```python
from build123d import *

# Parameters (mm, degrees)
CYLINDER081_R     = 13.5
CYLINDER081_DEPTH = 20
CYLINDER080_R     = 15.7
CYLINDER080_DEPTH = 14
CYLINDER083_R     = 11
CYLINDER083_DEPTH = 1
CYLINDER082_R     = 15
CYLINDER082_DEPTH = 1


with BuildPart() as internal_border:
    # Cylinder081 → Cylinder081 (new body)
    with BuildSketch(Plane.XY):
        Circle(CYLINDER081_R)
    extrude(amount=CYLINDER081_DEPTH)


with BuildPart() as adapter_tube_cut:
    # Cylinder080 → Cylinder080 (new body)
    with BuildSketch(Plane.XY):
        Circle(CYLINDER080_R)
    extrude(amount=CYLINDER080_DEPTH)

    # Cut023016: cut internal border
    add(internal_border.part, mode=Mode.SUBTRACT)


with BuildPart() as top_plate_hole:
    # Cylinder083 → Cylinder083 (new body)
    with BuildSketch(Plane.XY):
        Circle(CYLINDER083_R)
    extrude(amount=CYLINDER083_DEPTH)


with BuildPart() as eyepiece_adapter_fusion:
    # Cylinder082 → Cylinder082 (new body)
    with BuildSketch(Plane.XY):
        Circle(CYLINDER082_R)
    extrude(amount=CYLINDER082_DEPTH)

    # Cut023015: cut top plate hole
    add(top_plate_hole.part, mode=Mode.SUBTRACT)

    # Fusion057: union adapter tube cut
    add(adapter_tube_cut.part)


solid = eyepiece_adapter_fusion.part
```
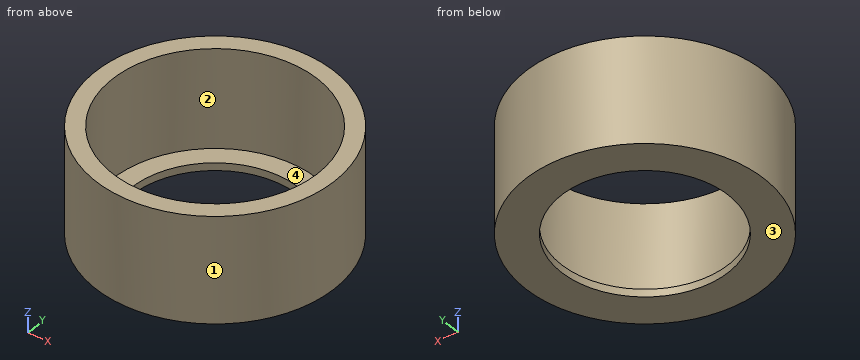
Verification items for the finished model (mm, model axes). Face numbers are marked on the shaded views. Coordinates: 2 decimals unless noted, no trailing zeros. Order: outer loops, then holes, each group sorted by start corner. A loop starts at its lowest first (then second) coordinate and runs counter-clockwise, first axis right, second up. Notation, with made-up numbers: (-21, 71.5) -> (12, 71.5) arc R21 cw to (12, 109.5) -> close; hole circle Ø4 at (56.25, -31.5). An arc over 180 degrees is marked (long way). Answer as CSV lines item,"result". Start each with the question number.
1) Cross-section at D-D, the plane y = -12. Record the boundary of the cut face in (x, z), then the cut area to 3 significant figures.
2) Gauge pin test, flat ends, axial feed: pin 1 Ø3 at (y, z) = (12.5, 2.5) entering from -X; pin 2 Ø8 at (y, z) = (-10, 7.5) entering from +X; pin 3 Ø2 at (x, z) = (8.5, 11.5) entering from +Y. Record the tip position at first contact, or that the pin passes through.
3) Cross-section at C-C, the plane z = 9. Record the boundary of the cut face in (x, y).
4) Release check for a two-part mould opening along X. For the marked faces 1, 2, 3 and 4 record: released by +X, released by -X, zero draft, split by the parting line, or undercut.
5) Cross-section at A-A, the plane y = 0. Record the boundary of the cut face in (x, z).
6) Material ranges on L1, parallel to Y at x = 0, z = 5.5; L2, parallel to Y at x = 0, z = 0.7; L3, parallel to Z at x = 7, y = -9, recorded low to high. Write a range as [from, to].
Conclusion:
1,outline,"(-10.12, 0) -> (10.12, 0) -> (10.12, 14) -> (6.18, 14) -> (6.18, 1) -> (-6.18, 1) -> (-6.18, 14) -> (-10.12, 14) -> close"
1,area,"123 mm²"
2,pin 1,"stops at x = -11.2"
2,pin 2,"stops at x = 14.51"
2,pin 3,"stops at y = 13.79"
3,outline,"circle Ø31.4 at (0, 0); hole circle Ø27 at (0, 0)"
4,face 1,"split by the parting line"
4,face 2,"undercut"
4,face 3,"zero draft"
4,face 4,"undercut"
5,outline,"(-15.7, 0) -> (-11, 0) -> (-11, 1) -> (-13.5, 1) -> (-13.5, 14) -> (-15.7, 14) -> close; (11, 0) -> (15.7, 0) -> (15.7, 14) -> (13.5, 14) -> (13.5, 1) -> (11, 1) -> close"
6,L1,"y = [-15.7, -13.5], [13.5, 15.7]"
6,L2,"y = [-15.7, -11], [11, 15.7]"
6,L3,"z = [0, 1]"
